from build123d import *

# Parameters (mm, degrees)
SKETCH_1_W                   = 40
SKETCH_1_H                   = 40
SKETCH_1_R                   = 7.5
EXTRUDE_1_DEPTH              = 3
SKETCH_23_W                  = 40
SKETCH_23_H                  = 40
SKETCH_23_R                  = 7.5
EXTRUDE_4_DEPTH              = 1.5
HOLE_WIZARD_M3_1_D           = 3.2
HOLE_WIZARD_M3_1_CBORE_D     = 6
HOLE_WIZARD_M3_1_CBORE_DEPTH = 4
F_3_0MM_1_D                  = 3
F_3_0MM_1_DEPTH              = 4
F_3_0MM_1_TIP                = 0.901290929
SKETCH_26_OUTSIDE_W          = 53.412
SKETCH_26_OUTSIDE_H          = 53.412
CUT_EXTRUDE_1_DEPTH          = 30.261749777
FILLET_2_R                   = 4
FILLET_3_R                   = 1
CHAMFER_1_SIZE               = 0.5


with BuildPart() as part:
    # 草图1 → 凸台-拉伸1 (new, symmetric)
    with BuildSketch(Plane.XY):
        Rectangle(SKETCH_1_W, SKETCH_1_H)
        Circle(SKETCH_1_R, mode=Mode.SUBTRACT)
    extrude(amount=EXTRUDE_1_DEPTH, both=True)

    # 草图23 → 凸台-拉伸4 (add)
    with BuildSketch(Plane.XY.offset(3)):
        Rectangle(SKETCH_23_W, SKETCH_23_H)
        Circle(SKETCH_23_R, mode=Mode.SUBTRACT)
    extrude(amount=EXTRUDE_4_DEPTH)

    # M3 六角圆柱头螺钉的柱形沉头孔1 (through all)
    with Locations(Plane(origin=(0, 0, -3), x_dir=(-1, 0, 0), z_dir=(0, 0, -1))):
        with Locations((-12, 0), (6, 10.392304845), (6, -10.392304845)):
            CounterBoreHole(HOLE_WIZARD_M3_1_D / 2, HOLE_WIZARD_M3_1_CBORE_D / 2, HOLE_WIZARD_M3_1_CBORE_DEPTH)

    # Ø3.0mm 暗销孔1
    with Locations(Plane.XY.offset(4.5)):
        with Locations((-12, 0), (6, 10.392304845), (6, -10.392304845)):
            Hole(F_3_0MM_1_D / 2, depth=F_3_0MM_1_DEPTH)
            with Locations((0, 0, -(F_3_0MM_1_DEPTH + F_3_0MM_1_TIP / 2))):  # 118° drill point
                Cone(0, F_3_0MM_1_D / 2, F_3_0MM_1_TIP, mode=Mode.SUBTRACT)

    # 草图26 outside → 切除-拉伸1 (cut, through all)
    with BuildSketch(Plane(origin=(0, 0, -3), x_dir=(-1, 0, 0), z_dir=(0, 0, -1))):
        Rectangle(SKETCH_26_OUTSIDE_W, SKETCH_26_OUTSIDE_H)
        Polygon((-17.320508076, 0), (-8.660254038, -15), (8.660254038, -15), (17.320508076, 0), (8.660254038, 15), (-8.660254038, 15), align=None, mode=Mode.SUBTRACT)
    extrude(amount=-CUT_EXTRUDE_1_DEPTH, mode=Mode.SUBTRACT)

    # 扫描1: sweep along a path in 草图44
    with BuildLine(Plane(origin=(0, 0, -1), x_dir=(-1, 0, 0), z_dir=(0, 0, -1))) as sweep_1_path:
        Line((-17.320508076, 0), (-8.660254038, -15))
        Line((-8.660254038, -15), (8.660254038, -15))
        Line((8.660254038, -15), (17.320508076, 0))
        Line((17.320508076, 0), (8.660254038, 15))
        Line((8.660254038, 15), (-8.660254038, 15))
        Line((-8.660254038, 15), (-17.320508076, 0))
    # 草图43 → 扫描1 (sweep)
    with BuildSketch(Plane(origin=(0, 0, 0), x_dir=(0, 0, -1), z_dir=(1, 0, 0))):
        Polygon((-1, 15), (1, 15), (0.636029766, 16), (-0.636029766, 16), align=None)
    sweep(path=sweep_1_path.line, transition=Transition.RIGHT)

    # 圆角2
    fillet_2_edges = [part.edges().sort_by_distance(p)[0] for p in [
        (-18.475208614, 0, 0),
        (-9.237604307, 16, 0),
        (-9.237604307, -16, 0),
        (9.237604307, 16, 0),
        (9.237604307, -16, 0),
        (18.475208614, 0, 0),
    ]]
    fillet(fillet_2_edges, radius=FILLET_2_R)

    # 圆角3
    fillet_3_edges = [part.edges().sort_by_distance(p)[0] for p in [
        (17.320508076, 0, -2),
        (8.660254038, -15, -2),
        (-8.660254038, -15, -2),
        (-17.320508076, 0, -2),
        (-8.660254038, 15, -2),
        (8.660254038, 15, -2),
        (8.660254038, 15, 2.75),
        (-8.660254038, 15, 2.75),
        (-17.320508076, 0, 2.75),
        (-8.660254038, -15, 2.75),
        (8.660254038, -15, 2.75),
        (17.320508076, 0, 2.75),
    ]]
    fillet(fillet_3_edges, radius=FILLET_3_R)

    # 倒角1
    chamfer_1_edges = [part.edges().sort_by_distance(p)[0] for p in [
        (-7.5, 0, -3),
        (-12.990381057, 7.5, -3),
        (12.990381057, 7.5, -3),
        (12.990381057, -7.5, -3),
        (0, -15, -3),
        (-12.990381057, -7.5, -3),
        (-7.5, 0, 4.5),
        (0, 15, -3),
        (8.582903769, 14.866025404, -3),
        (17.165807537, 0, -3),
        (8.582903769, -14.866025404, -3),
        (-8.582903769, -14.866025404, -3),
        (-17.165807537, 0, -3),
        (-8.582903769, 14.866025404, -3),
        (-12.990381057, 7.5, 4.5),
        (0, 15, 4.5),
        (12.990381057, -7.5, 4.5),
        (12.990381057, 7.5, 4.5),
        (-12.990381057, -7.5, 4.5),
        (0, -15, 4.5),
        (8.582903769, 14.866025404, 4.5),
        (17.165807537, 0, 4.5),
        (8.582903769, -14.866025404, 4.5),
        (-8.582903769, -14.866025404, 4.5),
        (-17.165807537, 0, 4.5),
        (-8.582903769, 14.866025404, 4.5),
    ]]
    chamfer(chamfer_1_edges, length=CHAMFER_1_SIZE)


solid = part.part
Here's how the part is built. I have some questions about the finished solid (model axes, mm). A direction names the side the tool comes from. Round coordinates to 2 decimals unless told otherwise and drop trailing zeros. Loops run counter-clockwise (first coordinate to the right, second up) from the corner with the lowest first, then second, coordinate; pieces in that order, holes last. Notation, with made-up numbers: M 77.5,29 L 94.5,29 A23 ccw 94.5,58 Z; hole C -16,61.5 d8. An arc over 180 degrees is marked long. Write each question's results on one line, items separated by ' | '. Start each with the question number.
(1) I want a section at A-A (x = 0). Please give me the cut outline in (y, z).
(2) I want a section at D-D (x = -14.5). Please give me the cut outline in (y, z).
(3) If I drill on probe 1 along X at (y, z) = (11.5, 2.25); probe 2 along Y at (x, z) = (-5.5, -2.25); probe 3 along X at (y, z) = (2.5, 0.5), over which ranges is the centre line in solid material (lowest first)? Write a range as from..to.
(4) On a 3-axis mill with a long thin cutter (end or side, diameter ignored), from which of +Z, -Z, +X, -X, +Y, -Y can I reach the whole of each face in a straight line? I mean faces 1 (the flat face through (0, -15, -2)), 2 (the cylindrical face through (-8.577, -14.87, -1.74)), 3 (the flat face through (13.05, -7.4, -1.76)), 4 (the cylindrical face through (-8.577, -14.87, 2.521)). Say none if no direction works.
(5) Thinking about a two-plate mould opening in Y: for faces 5 (the cylindrical face through (8.577, -14.87, 2.521)), 6 (the flat face through (0.125, 15.425, -0.845)), 7 (the cylindrical face through (-5.609, 13.367, -1.028)), which applies, pulls with the +Y half, pulls with the -Y half, needs draft (parallel to the pull), parting line crosses it, or undercut?
(6) I want a section at C-C (z = 2). Please give me the cut outline in (x, y), then the cut area to 3 significant figures.
(7) I want a section at B-B (z = -1.5). Please give me the cut outline in (x, y), then the cut area to 3 significant figures.
(8) Will these pins go through, and if not, where does the flat tip stop? P1, Ø4, axis at x = -6, z = -2, coming from the +Y side; P2, Ø3, axis at x = 12.5, y = -0.5, coming from the -Z side; P3, Ø0.8, axis at x = 1, z = -2, coming from the +Y side; P4, Ø1.2, axis at x = -3.5, z = -2, coming from the -Y side.
Solved:
1) outline: M -16,-0.64 L -15,-1 L -15,-2.5 L -14.5,-3 L -8,-3 L -7.5,-2.5 L -7.5,4 L -8,4.5 L -14.5,4.5 L -15,4 L -15,1 L -16,0.64 Z; M 7.5,-2.5 L 8,-3 L 14.5,-3 L 15,-2.5 L 15,-1 L 16,-0.64 L 16,0.64 L 15,1 L 15,4 L 14.5,4.5 L 8,4.5 L 7.5,4 Z
2) outline: M -6.89,-0.64 L -4.89,-1 L -4.89,-2.5 L -3.89,-3 L 3.89,-3 L 4.89,-2.5 L 4.89,-1 L 6.89,-0.64 L 6.89,0.64 L 4.89,1 L 4.89,4 L 3.89,4.5 L -3.89,4.5 L -4.89,4 L -4.89,1 L -6.89,0.64 Z
3) probe 1: x = -10.68..-7.15, -4.85..4.99, 7.01..10.68 | probe 2: y = -15..-13.35, -7.43..-5.1, 5.1..7.43, 13.35..15 | probe 3: x = -17.03..-7.07, 7.07..10.34, 13.66..17.03
4) face 1: -Z, +X, -X, -Y | face 2: -Z, -X, -Y | face 3: -Z, +X, -Y | face 4: +Z, -X, -Y
5) face 5: pulls with the -Y half | face 6: pulls with the +Y half | face 7: undercut
6) outline: M -17.03,-0.5 L -8.95,-14.5 A1 ccw -8.08,-15 L 8.08,-15 A1 ccw 8.95,-14.5 L 17.03,-0.5 A1 ccw 17.03,0.5 L 8.95,14.5 A1 ccw 8.08,15 L -8.08,15 A1 ccw -8.95,14.5 L -17.03,0.5 A1 ccw Z; hole C -12,0 d3; hole C -6,-10.39 d3.2; hole C -6,10.39 d3.2; hole C 0,0 d15; hole C 6,-10.39 d3; hole C 6,10.39 d3; hole C 12,0 d3.2 | area: 557 mm²
7) outline: M -17.03,-0.5 L -8.95,-14.5 A1 ccw -8.08,-15 L 8.08,-15 A1 ccw 8.95,-14.5 L 17.03,-0.5 A1 ccw 17.03,0.5 L 8.95,14.5 A1 ccw 8.08,15 L -8.08,15 A1 ccw -8.95,14.5 L -17.03,0.5 A1 ccw Z; hole C -6,-10.39 d6; hole C -6,10.39 d6; hole C 0,0 d15; hole C 12,0 d6 | area: 518 mm²
8) P1: stops at y = 16 | P2: stops at z = 1 | P3: stops at y = 15 | P4: stops at y = -15
